Geometry: final body of the model. Coordinates: model frame, mm. Face numbers are marked on the shaded views. A direction names the side the tool comes from. Coordinates: 2 decimals unless noted, no trailing zeros. Write each loop counter-clockwise with the first axis right and the second up, starting at its lowest first coordinate (ties: lowest second). Pieces come first, ordered by that corner, then holes.
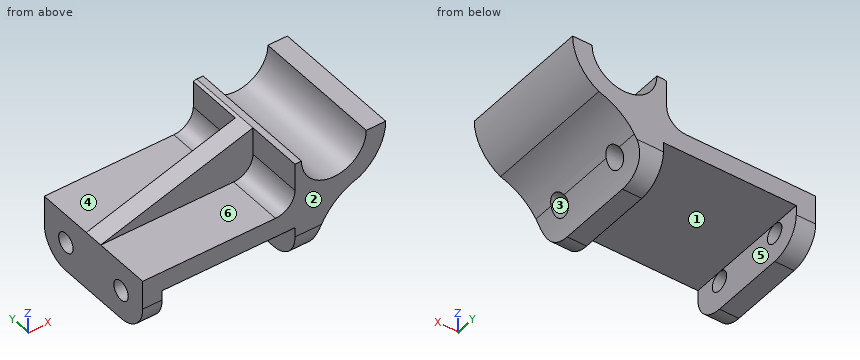
from build123d import *

# Parameters (mm, degrees)
F0_W      = 150
F0_H      = 65
F1_DEPTH  = 82
F10_W     = 82
F10_H     = 24
F2_DEPTH  = 82
F3_DEPTH  = 82
F4_DEPTH  = 82
F5_DEPTH  = 35
F7_DEPTH  = 35
F8_R      = 6
F12_R     = 6
F13_DEPTH = 150
F14_DEPTH = 150
F9_DEPTH  = 82


# Not quite as in the source:
# - a feature names something its author has since deleted; it is built from what else it names


with BuildPart() as f1:
    # F0 (on Front) → F1 (new body)
    with BuildSketch(Plane.XZ):
        with Locations((-16.9468223028, 32.5)):
            Rectangle(F0_W, F0_H)
    extrude(amount=F1_DEPTH)

    # F10 (on face) → F2 (cut)
    with BuildSketch(Plane.XZ.offset(82)):
        with BuildLine():
            ThreePointArc((20.002534413, 20.6353670047), (15.5702030299, 10.7379376133), (14.0531776972, 0))
            Line((14.0531776972, 0), (58.0531776972, 0))
            Line((58.0531776972, 0), (58.0531776972, 65))
            ThreePointArc((58.0531776972, 65), (53.7152597827, 48.9124515634), (41.8776017786, 37.1865571621))
            ThreePointArc((41.8776017786, 37.1865571621), (37.6930401765, 19.9858202792), (20.002534413, 20.6353670047))
        make_face()
        with Locations((-38.9468223028, 12)):
            Rectangle(F10_W, F10_H)
    extrude(amount=-F2_DEPTH, mode=Mode.SUBTRACT)

    # F11 (on face) → F3 (cut)
    with BuildSketch(Plane.XZ.offset(82)):
        Polygon((-91.9468223028, 36), (2.0531776972, 65), (-91.9468223028, 65), align=None)
    extrude(amount=-F3_DEPTH, mode=Mode.SUBTRACT)

    # F11 (on face) → F4 (cut)
    with BuildSketch(Plane.XZ.offset(82)):
        Polygon((-91.9468223028, 36), (2.0531776972, 65), (-91.9468223028, 65), align=None)
    extrude(amount=-F4_DEPTH, mode=Mode.SUBTRACT)

    # F11 (on face) → F5 (cut)
    with BuildSketch(Plane.XZ.offset(82)):
        with BuildLine():
            Line((2.0531776972, 48), (2.0531776972, 65))
            Line((2.0531776972, 65), (-91.9468223028, 36))
            Line((-91.9468223028, 36), (-9.9468223028, 36))
            ThreePointArc((-9.9468223028, 36), (-1.4615409285, 39.5147186258), (2.0531776972, 48))
        make_face()
    extrude(amount=-F5_DEPTH, mode=Mode.SUBTRACT)

    # F6 (on face) → F7 (cut)
    with BuildSketch(Plane(origin=(0, 0, 0), x_dir=(-1, 0, 0), z_dir=(0, 1, 0))):
        with BuildLine():
            Line((12, 36), (91.9468223028, 36))
            Line((91.9468223028, 36), (0, 64.3665728381))
            Line((0, 64.3665728381), (0, 48))
            ThreePointArc((0, 48), (3.5147186258, 39.5147186258), (12, 36))
        make_face()
    extrude(amount=-F7_DEPTH, mode=Mode.SUBTRACT)

    # F8 (on face) + F12 (on face) → F13 (cut)
    with BuildSketch(Plane(origin=(-91.9468223028, 0, 0), x_dir=(0, -1, 0), z_dir=(-1, 0, 0))):
        with Locations((18, 18)):
            Circle(F8_R)
        with Locations((64, 18)):
            Circle(F8_R)
    with BuildSketch(Plane(origin=(-91.9468223028, 0, 0), x_dir=(0, -1, 0), z_dir=(-1, 0, 0))):
        with Locations((18, 18)):
            Circle(F12_R)
    extrude(amount=-F13_DEPTH, mode=Mode.SUBTRACT)

    # F8 (on face) → F14 (cut)
    with BuildSketch(Plane(origin=(-91.9468223028, 0, 0), x_dir=(0, -1, 0), z_dir=(-1, 0, 0))):
        with BuildLine():
            Line((0, 0), (18, 0))
            ThreePointArc((18, 0), (5.2720779386, 5.2720779386), (0, 18))
            Line((0, 18), (0, 0))
        make_face()
        with BuildLine():
            ThreePointArc((82, 18), (76.7279220614, 5.2720779386), (64, 0))
            Line((64, 0), (82, 0))
            Line((82, 0), (82, 18))
        make_face()
    extrude(amount=-F14_DEPTH, mode=Mode.SUBTRACT)

    # F10 (on face) → F9 (cut)
    with BuildSketch(Plane.XZ.offset(82)):
        with BuildLine():
            ThreePointArc((41.8776017786, 37.1865571621), (29.4269949399, 30.9107323053), (20.002534413, 20.6353670047))
            ThreePointArc((20.002534413, 20.6353670047), (37.6930401765, 19.9858202792), (41.8776017786, 37.1865571621))
        make_face()
        with BuildLine():
            ThreePointArc((20.002534413, 20.6353670047), (15.5702030299, 10.7379376133), (14.0531776972, 0))
            Line((14.0531776972, 0), (58.0531776972, 0))
            Line((58.0531776972, 0), (58.0531776972, 65))
            ThreePointArc((58.0531776972, 65), (53.7152597827, 48.9124515634), (41.8776017786, 37.1865571621))
            ThreePointArc((41.8776017786, 37.1865571621), (37.6930401765, 19.9858202792), (20.002534413, 20.6353670047))
        make_face()
        with BuildLine():
            Line((46.0531776972, 65), (6.0531776972, 65))
            ThreePointArc((6.0531776972, 65), (12.5913823165, 50.2087841904), (27.9311842099, 45.0883679338))
            ThreePointArc((27.9311842099, 45.0883679338), (40.8443935069, 51.5382046192), (46.0531776972, 65))
        make_face()
    extrude(amount=-F9_DEPTH, mode=Mode.SUBTRACT)


solid = f1.part
Item 1: Pull-direction query (Z, two-part tool) for the marked faces 1, 2 and 3; classes: released by +Z, released by -Z, zero draft, split by the parting line, or undercut.
Derived:
face 1: released by -Z
face 2: zero draft
face 3: undercut
Item 2: Material intervals for probe 1 along Y at (x, z) = (-84.25, 18); probe 2 along Y at (x, z) = (4.5, 16.5); probe 3 along Z at (x, y) = (-85.5, -18), sorted ascending.
Derived:
probe 1: y = -82 to -70, -58 to -24, -12 to 0
probe 2: y = -81.94 to -69.81, -58.19 to -23.81, -12.19 to -0.06
probe 3: z = 0 to 12, 24 to 36
Item 3: Section B-B, the plane y = -41. Output: boundary loops of the cut face in (x, z), plus the area to 3 significant figures.
Derived:
outline: (-91.95, 0) - (-79.95, 0) - (-79.95, 24) - (2.05, 24) - (2.05, 0) - (14.05, 0) arc R38.76 cw to (41.88, 37.19) arc R32 ccw to (58.05, 65) - (46.05, 65) arc R20 cw to (6.05, 65) - (2.05, 65) - (-91.95, 36) - close
area: 4,300 mm2
Item 4: Section D-D, the plane y = -28. Output: boundary loops of the cut face in (x, z).
Derived:
outline: (-91.95, 0) - (-79.95, 0) - (-79.95, 24) - (2.05, 24) - (2.05, 0) - (14.05, 0) arc R38.76 cw to (41.88, 37.19) arc R32 ccw to (58.05, 65) - (46.05, 65) arc R20 cw to (6.05, 65) - (2.05, 65) - (0, 64.37) - (0, 48) arc R12 cw to (-12, 36) - (-91.95, 36) - close
Item 5: Section A-A, the plane z = 60. Output: boundary loops of the cut face in (x, y).
Derived:
outline: (-14.15, -47) - (2.05, -47) - (2.05, -82) - (6.69, -82) - (6.69, 0) - (0, 0) - (0, -35) - (-14.15, -35) - close; (45.42, -82) - (57.66, -82) - (57.66, 0) - (45.42, 0) - close
Item 6: Pin query (flat end, axial travel): pin 1 (10 mm diameter, centred on x = -73, y = -50, fed in from -Z); pin 2 (8.5 mm diameter, centred on y = -72, z = 58, fed in from -X); pin 3 (12 mm diameter, centred on y = -48, z = 46, fed in from +X). Return the tip coordinate at first contact, or that it passes through.
Derived:
pin 1: stops at z = 24
pin 2: stops at x = 2.05
pin 3: stops at x = 55.29
Item 7: Section C-C, the plane y = -62.5. Output: boundary loops of the cut face in (x, z), plus the area to 3 significant figures.
Derived:
outline: (-91.95, 0) - (-79.95, 0) - (-79.95, 12.19) - (-91.95, 12.19) - close; (-91.95, 23.81) - (-79.95, 23.81) - (-79.95, 24) - (2.05, 24) - (2.05, 23.81) - (22.23, 23.81) arc R38.76 cw to (41.88, 37.19) arc R32 ccw to (58.05, 65) - (46.05, 65) arc R20 cw to (6.05, 65) - (2.05, 65) - (2.05, 48) arc R12 cw to (-9.95, 36) - (-91.95, 36) - close; (2.05, 0) - (14.05, 0) arc R38.76 cw to (16.02, 12.19) - (2.05, 12.19) - close
area: 2,630 mm2
Item 8: Set-up query: the marked faces 4, 5 and 6. Return all of +Z, -Z, +X, -X, +Y, -Y with unobstructed straight access to the full face (end or side cutting, diameter ignored); none if empty.
Derived:
face 4: +Z, -X, +Y
face 5: -Z, +Y, -Y
face 6: +Z, -X, -Y
